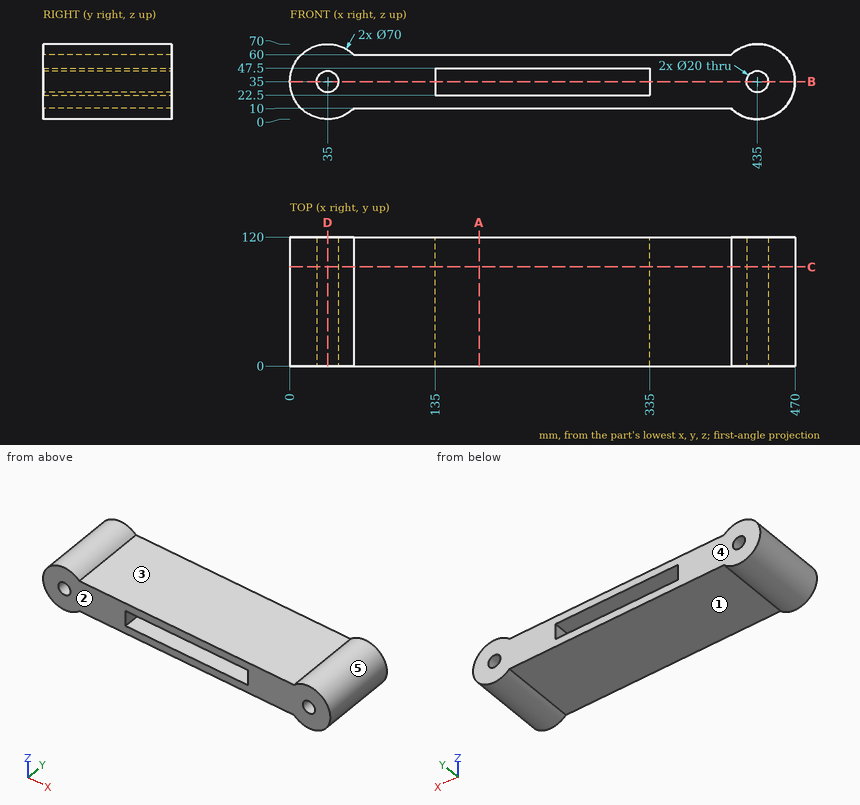
Here's the drawing with two shaded views (mm, measured from the low corner). I have some questions. A direction names the side the tool comes from. Round coordinates to 2 decimals unless told otherwise and drop trailing zeros. Order: outer loops, then holes, each group sorted by start corner. A loop starts at its lowest first (then second) coordinate and runs counter-clockwise, first axis right, second up. Notation, with made-up numbers: (11.5, 40) -> (44.5, 40) arc R21 ccw to (44.5, 45) -> close; hole circle Ø7 at (-39, 18.25). An arc over 180 degrees is marked (long way). Use a Markdown table: item, result. Add a question column.
(1) If we mould it in two halves opening along X, with no side actions, what happens to the marked faces 4 and 5? For each: released by +X, released by -X, zero draft, split by the parting line, or undercut.
(2) For the marked faces 1, 2 and 3, which set-ups out of +Z, -Z, +X, -X, +Y, -Y let a thin tool reach every point of the face, with its end or its side?
(3) Suppose I cut it at A-A, the plane x = 176. Please give me the cut outline in (y, z).
(4) Suppose I cut it at B-B, the plane z = 35. Please give me the cut outline in (x, y).
(5) Suppose I cut it at C-C, the plane y = 92.5. Please give me the cut outline in (x, z), and give its area (3 significant figures).
(6) For pin 1 Ø1 at (x, y) = (198, 38.5) entering from +Z; pin 2 Ø4 at (y, z) = (52, 8) entering from -X; pin 3 Ø8 at (y, z) = (94.5, 26.5) entering from +X, each with a flat end and sliding along its axis, tell me the tip position at first contact or that it passes through.
(7) Suppose I cut it at D-D, the plane x = 35. Please give me the cut outline in (y, z).
(8) I need wall thicknesses on line 1 along X through (y, z) = (115, 40.5); line 2 along Z through (x, y) = (137, 58); line 3 along Z through (x, y) = (435, 59.5). Which ranges of each line are inside material? Lowest first, please.
Verdict:
| question | item | result |
|---|---|---|
| 1 | face 4 | zero draft |
| 1 | face 5 | undercut |
| 2 | face 1 | -Z, +Y, -Y |
| 2 | face 2 | +Z, -Z, +X, -X, -Y |
| 2 | face 3 | +Z, +Y, -Y |
| 3 | outline | (0, 10) -> (120, 10) -> (120, 22.5) -> (0, 22.5) -> close; (0, 47.5) -> (120, 47.5) -> (120, 60) -> (0, 60) -> close |
| 4 | outline | (0, 0) -> (25, 0) -> (25, 120) -> (0, 120) -> close; (45, 0) -> (135, 0) -> (135, 120) -> (45, 120) -> close; (335, 0) -> (425, 0) -> (425, 120) -> (335, 120) -> close; (445, 0) -> (470, 0) -> (470, 120) -> (445, 120) -> close |
| 5 | outline | (59.49, 10) -> (410.51, 10) arc R35 ccw (long way) to (410.51, 60) -> (59.49, 60) arc R35 ccw (long way) to start; hole circle Ø20 at (35, 35); hole (135, 22.5) -> (335, 22.5) -> (335, 47.5) -> (135, 47.5) -> close; hole circle Ø20 at (435, 35) |
| 5 | area | 18,900 mm2 |
| 6 | pin 1 | z = 60 |
| 6 | pin 2 | x = 10.51 |
| 6 | pin 3 | x = 469.71 |
| 7 | outline | (0, 0) -> (120, 0) -> (120, 25) -> (0, 25) -> close; (0, 45) -> (120, 45) -> (120, 70) -> (0, 70) -> close |
| 8 | line 1 | 0.43 to 26.65, 43.35 to 135, 335 to 426.65, 443.35 to 469.57 |
| 8 | line 2 | 10 to 22.5, 47.5 to 60 |
| 8 | line 3 | 0 to 25, 45 to 70 |
